Job drawing, mm, ordinate dimensions from the low corner. One solid piece. Round coordinates to 2 decimals unless told otherwise and drop trailing zeros. Loops run counter-clockwise (first coordinate to the right, second up) from the corner with the lowest first, then second, coordinate; pieces in that order, holes last.
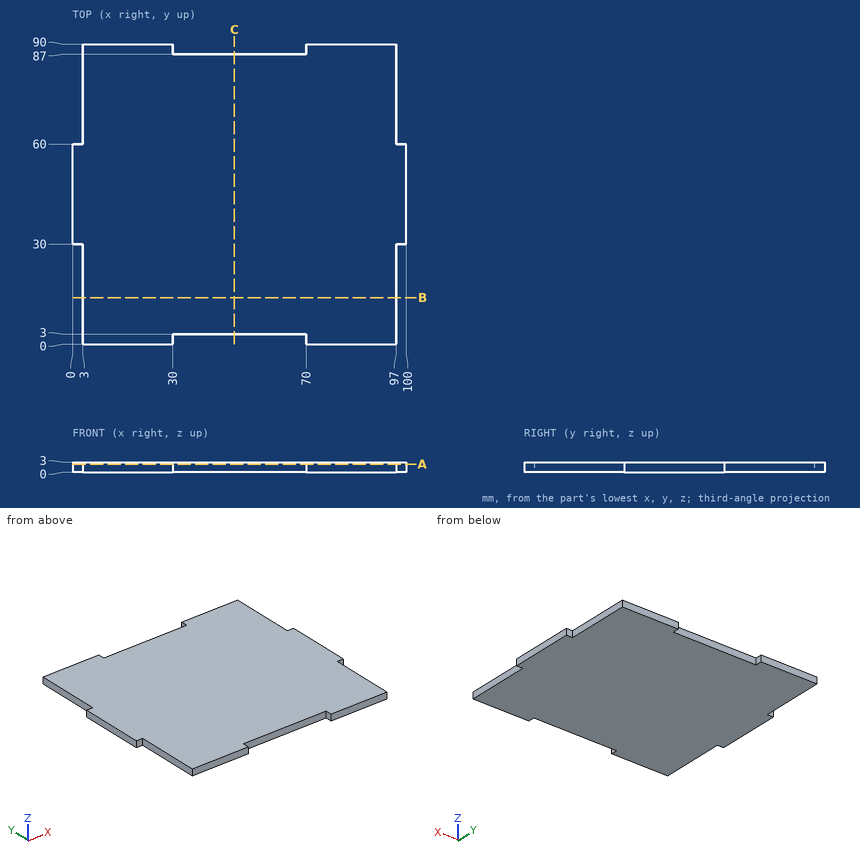
Item 1: Flat gauge pins, fed straight in: P1, Ø1.5, axis at x = 55.5, z = 1, coming from the -Y side; P2, Ø1.5, axis at y = 70.5, z = 1.5, coming from the -X side; P3, Ø0.9, axis at y = 20, z = 1, coming from the +X side. Where does each tip first touch, or does it go through?
Answers follow:
P1: stops at y = 3
P2: stops at x = 3
P3: stops at x = 97
Item 2: Cut at C-C, the plane x = 48.5. Give the cut face in (y, z).
Answers follow:
outline: (3, 0) - (87, 0) - (87, 3) - (3, 3) - close
Item 3: Cut at B-B, the plane y = 14. Give the cut face in (x, z), plus the area to 3 significant figures.
Answers follow:
outline: (3, 0) - (97, 0) - (97, 3) - (3, 3) - close
area: 282 mm2
Item 4: Cut at A-A, the plane z = 2.45. Give the cut face in (x, y), plus the area to 3 significant figures.
Answers follow:
outline: (0, 30) - (3, 30) - (3, 0) - (30, 0) - (30, 3) - (70, 3) - (70, 0) - (97, 0) - (97, 30) - (100, 30) - (100, 60) - (97, 60) - (97, 90) - (70, 90) - (70, 87) - (30, 87) - (30, 90) - (3, 90) - (3, 60) - (0, 60) - close
area: 8,400 mm2
Item 5: Probe line 1 (X direction, y = 65.5, z = 0.3); line 2 (Y direction, x = 55.5, z = 0.5). List the from-to ranges inside material, lowest first.
Answers follow:
line 1: x = 3 to 97
line 2: y = 3 to 87
